```python
from build123d import *

# Parameters (mm, degrees)
F1_DEPTH = 40
F2_DEPTH = 15
F3_DEPTH = 5
F5_R     = 5


with BuildPart() as f1:
    # F0 (on Front) → F1 (new body, symmetric)
    with BuildSketch(Plane.XZ):
        Polygon((-60, -10), (60, -10), (60, 10), (40, 10), (-60, 10), align=None)
    extrude(amount=F1_DEPTH, both=True)

    # F0 (on Front) → F2 (join, symmetric)
    with BuildSketch(Plane.XZ):
        with BuildLine():
            Line((40, 10), (60, 10))
            Line((60, 10), (60, 20))
            ThreePointArc((60, 20), (64.393398, 30.606602), (75, 35))
            Line((75, 35), (84.064805, 35))
            Line((84.064805, 35), (84.064805, 55))
            Line((84.064805, 55), (75, 55))
            ThreePointArc((75, 55), (50.251263, 44.748737), (40, 20))
            Line((40, 20), (40, 10))
        make_face()
    extrude(amount=F2_DEPTH, both=True)

    # F0 (on Front) → F3 (join, symmetric)
    with BuildSketch(Plane.XZ):
        with BuildLine():
            add(Edge.make_bspline(
                [(-60, 10), (-55.525135, 51.721793), (7.100719, 55.106737), (75, 55)],
                knots=[0, 0, 0, 0, 142.302495, 142.302495, 142.302495, 142.302495], degree=3))
            Line((-60, 10), (40, 10))
            Line((40, 10), (40, 20))
            ThreePointArc((40, 20), (50.251263, 44.748737), (75, 55))
        make_face()
    extrude(amount=F3_DEPTH, both=True)

    # F0 (on Front) → F4 (revolve)
    with BuildSketch(Plane.XZ):
        Polygon((84.064805, 59.669833), (84.064805, 55), (84.064805, 35), (84.064805, 29.669833), (114.064805, 29.669833), (114.064805, 59.669833), align=None)
    revolve(axis=Axis((84.064805, 0, 44.669833), (0, 0, 1)))

    # F5
    f5_edges = [f1.edges().sort_by_distance(p)[0] for p in [
        (-60, -40, 0),
        (60, -40, 0),
        (60, 40, 0),
        (-60, 40, 0),
    ]]
    fillet(f5_edges, radius=F5_R)


solid = f1.part
```
CAD build for the part. Positions are in the model's coordinates, mm. A direction names the side the tool comes from. Give positions to 0.01 mm unless a question says otherwise; leave off trailing zeros. Write each loop counter-clockwise with the first axis right and the second up, starting at its lowest first coordinate (ties: lowest second). Pieces come first, ordered by that corner, then holes. Notation, with made-up numbers: M 42.5,60 L 95.5,60 A18 ccw 95.5,77 Z; hole C 18.25,14 d8. An arc over 180 degrees is marked long. Return JSON: item names as keys, results as strings. Group by question number.
(1) Flat gauge pins, fed straight in: pin 1 Ø13.5 at (x, z) = (-17.5, 43) entering from -Y; pin 2 Ø17 at (x, y) = (83.5, 10) entering from -Z; pin 3 Ø3 at (y, z) = (-8, 14) entering from -X. Where does each tip first touch, or does it go through?
(2) 3-axis set-ups, long thin cutter, end or side, ignore diameter. For faces 1 (the face through (-2, 5, 28)), 2 (the face through (-2, -5, 28)), 3 (the face through (-60, 0, 0)): which of +Z, -Z, +X, -X, +Y, -Y reach the whole face in a straight line?
(3) Band-saw the part on B-B (y = 9). Give the cut face in (x, z).
(4) Band-saw the part on A-A (z = 6). Give the cut face in (x, y).
(5) Drill centre lines: L1, parallel to Z at x = 15, y = -34; L2, parallel to X at y = 33, z = 8; L3, parallel to Y at x = 25, z = 35. Where is each one in solid material? Low to high. Write a range as [from, to].
Entries:
{
 "1": {"pin 1": "stops at y = -5", "pin 2": "stops at z = 29.67", "pin 3": "stops at x = 40"},
 "2": {"face 1": "+Z, -X, +Y", "face 2": "+Z, -X, -Y", "face 3": "+Z, -Z, -X, +Y, -Y"},
 "3": {"outline": "M -60,-10 L 60,-10 L 60,20 A15 cw 63.53,29.67 L 112.68,29.67 L 112.68,59.67 L 55.45,59.67 L 55.45,49.03 A35 ccw 40,20 L 40,10 L -60,10 Z"},
 "4": {"outline": "M -60,-35 A5 ccw -55,-40 L 55,-40 A5 ccw 60,-35 L 60,35 A5 ccw 55,40 L -55,40 A5 ccw -60,35 Z"},
 "5": {"L1": "z = [-10, 10]", "L2": "x = [-60, 60]", "L3": "y = [-5, 5]"}
}
